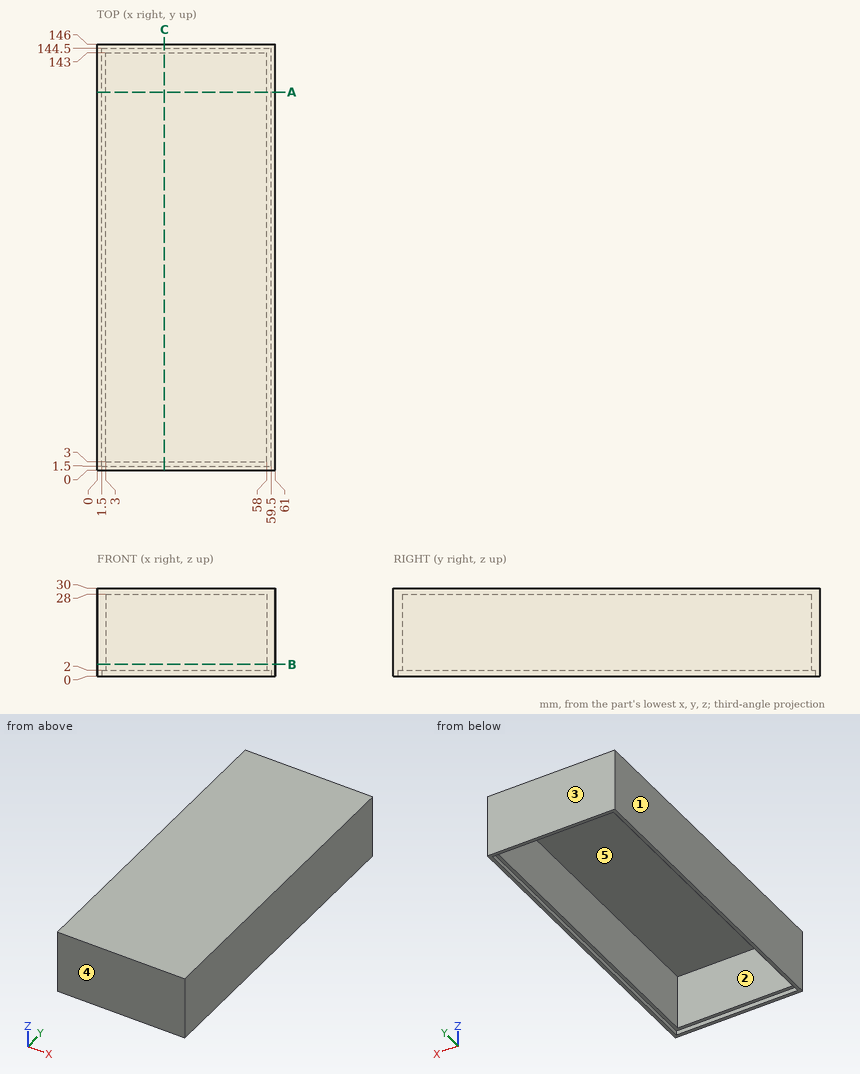
Could you check a few things on this drawing? It's one solid part, dimensions in mm from its lowest x, y, z. A direction names the side the tool comes from. Coordinates: 2 decimals unless noted, no trailing zeros. Order: outer loops, then holes, each group sorted by start corner. A loop starts at its lowest first (then second) coordinate and runs counter-clockwise, first axis right, second up.
1) Will this pin go through, and if not, where does the flat tip stop? pin 1 (6 mm diameter, centred on x = 53.5, y = 106, fed in from -Z).
2) We'd pull the mould along X, two halves only. Please class the marked faces 1, 2 and 3: +X half, -X half, draft (parallel to the pull), parting line (faces both ways), or undercut.
3) Imagine slicing it at C-C on x = 23. List the corners of the cut face in (y, z) for me, and give its area (3 significant figures).
4) Imagine slicing it at A-A on y = 129.5. List the corners of the cut face in (x, z) for me, and give its area (3 significant figures).
5) Which directions (+Z, -Z, +X, -X, +Y, -Y) give clear straight access to the entire face, cutting with the end or side of a thin tool? Please do the marked faces 4 and 5.
6) I need wall thicknesses on line 1 (Y direction, x = 33.5, z = 20.25); line 2 (X direction, y = 100, z = 8); line 3 (Y direction, x = 38, z = 1.75). Which ranges of each line are inside material? Lowest first, please.
7) Imagine slicing it at B-B on z = 4. List the corners of the cut face in (x, y) for me.
Response values:
1. pin 1: stops at z = 28
2. face 1: -X half
2. face 2: undercut
2. face 3: draft
3. outline: (0, 0) - (1.5, 0) - (1.5, 2) - (3, 2) - (3, 28) - (143, 28) - (143, 2) - (144.5, 2) - (144.5, 0) - (146, 0) - (146, 30) - (0, 30) - close
3. area: 454 mm2
4. outline: (0, 0) - (1.5, 0) - (1.5, 2) - (3, 2) - (3, 28) - (58, 28) - (58, 2) - (59.5, 2) - (59.5, 0) - (61, 0) - (61, 30) - (0, 30) - close
4. area: 284 mm2
5. face 4: +Z, -Z, +X, -X, -Y
5. face 5: -Z
6. line 1: y = 0 to 3, 143 to 146
6. line 2: x = 0 to 3, 58 to 61
6. line 3: y = 0 to 1.5, 144.5 to 146
7. outline: (0, 0) - (61, 0) - (61, 146) - (0, 146) - close; hole (3, 3) - (58, 3) - (58, 143) - (3, 143) - close
